Autodesk Inventor part; units mm, degrees
ref_plane "YZ Plane" through (0, 0, 0) normal (1, 0, 0) x (0, 1, 0)
ref_plane "XZ Plane" through (0, 0, 0) normal (0, 1, 0) x (-1, 0, 0)
ref_plane "XY Plane" through (0, 0, 0) normal (0, 0, 1) x (1, 0, 0)
sketch "Sketch1" plane through (0, 0, 0) normal (0, 0, 1) x (1, 0, 0)
  line L0 (-25, 25) -> (25, 25)
  line L1 (25, 25) -> (25, -25)
  line L2 (25, -25) -> (-25, -25)
  line L3 (-25, -25) -> (-25, 25)
  point P0 (0, 0)
  dimension "d0" = 50
  dimension "d1" = 25
  dimension "d2" = 25
  dimension "d3" = 25
extrude "Extrusion1" add sketch "Sketch1" along normal blind 350
sketch "Sketch2" plane through (-25, 25, 0) normal (0, 1, 0) x (1, 0, 0)
  line L0 (50, -350) -> (0, -350)
  line L1 (50, 0) -> (50, -350)
  line L2 (0, -350) -> (50, -350)
  line L3 (50, -350) -> (50, -320)
  line L4 (50, -320) -> (0, -320)
  line L5 (0, -320) -> (0, -350)
  point P0 (25, 0)
  dimension "d6" = 30
extrude "Extrusion2" add sketch "Sketch2" along normal blind 300
sketch "Sketch3" plane through (0, 0, 350) normal (0, 0, 1) x (1, 0, 0)
  line L0 (-25, 325) -> (25, 325)
  line L1 (25, -25) -> (25, 325)
  point P0 (0, 0)
  point P1 (0, 255)
  dimension "d9" = 70
  dimension "d10" = 25
hole "Hole1" at (0, 255, 350) direction (0, 0, -1) diameter 10.917 end through all
sketch "Sketch6" plane through (25, -25, 0) normal (1, 0, 0) x (0, 0, -1)
  line L0 (-75, 2.5) -> (-30, 2.5)
  line L1 (-30, 2.5) -> (-30, 47.5)
  line L2 (-30, 47.5) -> (-75, 47.5)
  line L3 (-75, 47.5) -> (-75, 2.5)
  line L4 (0, 50) -> (0, 0)
  line L5 (0, 0) -> (-350, 0)
  point P0 (0, 25)
  dimension "d36" = 45
  dimension "d37" = 45
  dimension "d38" = 30
  dimension "d39" = 2.5
extrude "Extrusion3" cut sketch "Sketch6" against normal blind 50
sketch "Sketch7" plane through (-25, -25, 0) normal (0, -1, 0) x (1, 0, 0)
  line L0 (50, 0) -> (0, 0)
  line L1 (50, 0) -> (50, 350)
  point P0 (25, 0)
  point P1 (25, 102)
  dimension "d42" = 102
  dimension "d43" = 25
hole "Hole4" at (0, -25, 102) direction (0, 1, 0) diameter 11.835 end through all
sketch "Sketch8" plane through (-25, -25, 0) normal (0, -1, 0) x (1, 0, 0)
  line L0 (2.5, 124) -> (47.5, 124)
  line L1 (47.5, 124) -> (47.5, 79)
  line L2 (47.5, 79) -> (2.5, 79)
  line L3 (2.5, 79) -> (2.5, 124)
  line L4 (50, 0) -> (0, 0)
  line L5 (0, 0) -> (0, 350)
  point P0 (25, 0)
  dimension "d51" = 45
  dimension "d52" = 45
  dimension "d53" = 79
  dimension "d54" = 2.5
extrude "Extrusion4" cut sketch "Sketch8" against normal blind 50
sketch "Sketch9" plane through (25, -25, 0) normal (1, 0, 0) x (0, 0, -1)
  line L0 (0, 50) -> (0, 0)
  line L1 (0, 0) -> (-350, 0)
  point P0 (0, 25)
  point P1 (-52.5, 25)
  dimension "d57" = 52.5
  dimension "d58" = 25
hole "Hole5" at (25, 0, 52.5) direction (-1, 0, 0) diameter 11.835 end through all
properties part number "brazo"
CAD build for the part. Positions are in the model's coordinates, mm. A direction names the side the tool comes from. Round coordinates to 2 decimals unless told otherwise and drop trailing zeros. Write each loop counter-clockwise with the first axis right and the second up, starting at its lowest first coordinate (ties: lowest second). Pieces come first, ordered by that corner, then holes.
(1) Slice it at D-D, the plane y = 154.5. Write the cut outline in (x, z), and give its area (3 significant figures).
(2) 3-axis set-ups, long thin cutter, end or side, ignore diameter. For faces 5 (the face through (0, 0, 124)), 6 (the face through (0, 152, 350)), 7 (the face through (0, -22.5, 53)), 8 (the face through (0, 25, 158)): which of +Z, -Z, +X, -X, +Y, -Y reach the whole face in a straight line?
(3) Slice it at B-B, the plane y = 255. Write the cut outline in (x, z), and give its area (3 significant figures).
(4) Slice it at C-C, the plane z = 188. Write the cut outline in (x, y).
(5) Probe line 1 along Z through (x, y) = (20, -7); line 2 along Y through (x, z) = (0, 338.5); line 3 along X through (y, z) = (255, 335). List the from-to ranges inside material, lowest first.
(6) Slice it at A-A, the plane x = -16. Write the cut outline in (y, z).
(7) Mould opens along X. For faces 1 (the face through (0, 0, 75)), 2 (the face through (-25, 20, 252)), 3 (the face through (0, 0, 79)), 4 (the face through (-22.5, 0, 101)) say: pulls with the +X half, pulls with the -X half, needs draft (parallel to the pull), parting line crosses it, or undercut.
(8) Drop flat-ended pins along their axis: P1, Ø1.5, axis at x = 1.5, z = 216, coming from the +Y side; P2, Ø2, axis at x = 16, y = 262.5, coming from the -Z side. Give the stop position or say it passes through.
From the geometry:
1. outline: (-25, 320) - (25, 320) - (25, 350) - (-25, 350) - close
1. area: 1,500 mm2
2. face 5: +Y, -Y
2. face 6: +Z, +X, -X, +Y, -Y
2. face 7: +X, -X
2. face 8: -Z, +X, -X, +Y
3. outline: (-25, 320) - (-5.46, 320) - (-5.46, 350) - (-25, 350) - close; (5.46, 320) - (25, 320) - (25, 350) - (5.46, 350) - close
3. area: 1,170 mm2
4. outline: (-25, -25) - (25, -25) - (25, 25) - (-25, 25) - close
5. line 1: z = 0 to 30, 75 to 79, 124 to 350
5. line 2: y = -25 to 249.54, 260.46 to 325
5. line 3: x = -25 to -5.46, 5.46 to 25
6. outline: (-25, 0) - (25, 0) - (25, 79) - (-25, 79) - close; (-25, 124) - (25, 124) - (25, 320) - (325, 320) - (325, 350) - (-25, 350) - close; hole (-22.5, 30) - (22.5, 30) - (22.5, 75) - (-22.5, 75) - close
7. face 1: needs draft
7. face 2: pulls with the -X half
7. face 3: undercut
7. face 4: undercut
8. P1: stops at y = 25
8. P2: stops at z = 320
